from build123d import *

# Parameters (mm, degrees)
SWEEP_THIN1_PROFILE_R     = 3.175
SWEEP_THIN1_PROFILE_R_2   = 2.175
BOSS_EXTRUDE1_OUTLINE_R   = 3.175
BOSS_EXTRUDE1_OUTLINE_R_2 = 2.175
BOSS_EXTRUDE1_DEPTH       = 5.033072262
BOSS_EXTRUDE1_START       = 3
BOSS_EXTRUDE1_2_DEPTH     = 8


with BuildPart() as part:
    # Sweep-Thin1: sweep along a curve in space
    with BuildLine() as sweep_thin1_path:
        Line((0, 0, 0), (0, 41.3, 0))
        Line((0, 41.3, 0), (0, 52.485381189, 0))
        ThreePointArc((8.731710823, 62.485381189, -4.874138499), (2.557458889, 59.556449001, -1.427602114), (0, 52.485381189, 0))
        Line((8.731710823, 62.485381189, -4.874138499), (26.239628077, 62.485381189, -14.647253442))
        ThreePointArc((26.239628077, 62.485381189, -14.647253442), (32.596698174, 65.949204532, -18.875029244), (33.90761411, 73.906143624, -21.166997899))
        Line((32.091284349, 81.948727145, -21.730096286), (33.90761411, 73.906143624, -21.166997899))
    # Sweep-Thin1 profile (on start of the path) → Sweep-Thin1 (sweep)
    with BuildSketch(Plane.ZX):
        Circle(SWEEP_THIN1_PROFILE_R)
        Circle(SWEEP_THIN1_PROFILE_R_2, mode=Mode.SUBTRACT)
    sweep(path=sweep_thin1_path.line)

    # Boss-Extrude1: read off the stored shape, not the designer's step
    # Boss-Extrude1 outline → Boss-Extrude1 (add)
    with BuildSketch(Plane(origin=(-16.302656388, 72.187043596, -5.054148045), x_dir=(0.9755496373305654, 0.2192425074835292, -0.015350179690706331), z_dir=(-0.21977921899989167, 0.973167297783081, -0.06813593340796047))):
        with Locations((49.606846115, 15.953433297)):
            Circle(BOSS_EXTRUDE1_OUTLINE_R)
        with Locations((49.606846115, 15.953433297)):
            Circle(BOSS_EXTRUDE1_OUTLINE_R_2, mode=Mode.SUBTRACT)
    extrude(amount=BOSS_EXTRUDE1_DEPTH)

    # Boss-Extrude1 2 outline → Boss-Extrude1 2 (cut)
    with BuildSketch(Plane(origin=(0, 0, 0), x_dir=(0.9092183851510403, -0.07176325268657005, -0.4100877511791569), z_dir=(0.41631950242972593, 0.156726908876634, 0.8956085908088649)).offset(BOSS_EXTRUDE1_START)):
        with BuildLine():
            ThreePointArc((30.991714154, 89.351616158), (32.537128586, 89.718539367), (34.090261078, 90.051282317))
            Line((34.090261078, 90.051282317), (35, 90.235713443))
            Line((35, 90.235713443), (35, 90.350121944))
            Line((35, 90.350121944), (34.072560393, 90.119086943))
            Line((34.072560393, 90.119086943), (30.991714154, 89.351616158))
        make_face()
        with BuildLine():
            ThreePointArc((27.927036801, 88.515957727), (29.454766368, 88.950690302), (30.991714154, 89.351616158))
            Line((30.991714154, 89.351616158), (27.910868159, 88.584144334))
            Line((27.910868159, 88.584144334), (27, 88.357237456))
            Line((27, 88.357237456), (27, 88.241069912))
            Line((27, 88.241069912), (27.927036801, 88.515957727))
        make_face()
    extrude(amount=BOSS_EXTRUDE1_2_DEPTH, mode=Mode.SUBTRACT)


solid = part.part
Source: CAD feature listing. Evaluate the final solid. Frame: model axes, mm. A direction names the side the tool comes from. Round coordinates to 2 decimals unless told otherwise and drop trailing zeros. Loops run counter-clockwise (first coordinate to the right, second up) from the corner with the lowest first, then second, coordinate; pieces in that order, holes last.
Q1. Access query for faces 5 (the face through (28.636, 86.302, -21.723)), 6 (the face through (-3.1, 26.61, -0.69)). Directions: +Z, -Z, +X, -X, +Y, -Y. A direction counts if a zero-diameter tool reaches every point of the face in a straight line with its end or side. Return the directions, or none.
Q2. Section A-A, the plane y = 34. Return loops of the section in (x, z) (3 decimals).
Q3. Ray query, line 1 (Z direction, x = -0.5, y = 45.5); line 2 (Y direction, x = 15, z = -7.75); line 3 (X direction, y = 23, z = -0.75). Return the intervals inside material, ascending.
Q4. First-contact query: P1, Ø5, axis at x = 30.5, y = 60, coming from the -Z side. Flat tip, straight axial feed; report the tip coordinate or a pass-through.
Q5. Mould query, pull axis Y, two halves, no side actions, for faces 1 (the face through (-2.123, 26.61, -0.471)), 2 (the face through (17.58, 64.66, -9.89)), 3 (the face through (32.69, 87.08, -23.74)), 4 (the face through (17.56, 65.66, -9.91)). Classes: pulls with the +Y half, pulls with the -Y half, needs draft (parallel to the pull), parting line crosses it, or undercut.
Solutions:
1. face 5: -Z, -X, +Y
1. face 6: -Y
2. outline: circle Ø6.35 at (0, 0); hole circle Ø4.35 at (0, 0)
3. line 1: z = -3.14 to -2.12, 2.12 to 3.14
3. line 2: y = 59.36 to 60.38, 64.59 to 65.61
3. line 3: x = -3.09 to -2.04, 2.04 to 3.09
4. P1: stops at z = -20.32
5. face 1: needs draft
5. face 2: undercut
5. face 3: pulls with the +Y half
5. face 4: parting line crosses it
